```python
from build123d import *

# Parameters (mm, degrees)
SKETCH022_R             = 2.5
PAD022_DEPTH            = 10
SKETCH023_R             = 1.5
PAD023_DEPTH            = 10
SKETCH024_W             = 8
SKETCH024_H             = 14
PAD024_DEPTH            = 10
SKETCH025_W             = 5
SKETCH025_H             = 2
PAD025_DEPTH            = 10
BODY009_PLACEMENT_ANGLE = 90


with BuildPart() as part:
    # Sketch022 → Pad022 (new body)
    with BuildSketch(Plane.XZ):
        Circle(SKETCH022_R)
    extrude(amount=PAD022_DEPTH)

    # Sketch023 (on Face3 of Pad022) → Pad023 (join)
    with BuildSketch(Plane.XZ.offset(10)):
        Circle(SKETCH023_R)
    extrude(amount=PAD023_DEPTH)

    # Sketch024 (on Face2 of Pad023) → Pad024 (join)
    with BuildSketch(Plane(origin=(0, 0, 0), x_dir=(1, 0, 0), z_dir=(0, 1, 0))):
        Rectangle(SKETCH024_W, SKETCH024_H)
    extrude(amount=PAD024_DEPTH)

    # Sketch025 (on Face5 of Pad024) → Pad025 (join)
    with BuildSketch(Plane(origin=(0, 10, 0), x_dir=(1, 0, 0), z_dir=(0, 1, 0))):
        with Locations((0, 4.5)):
            Rectangle(SKETCH025_W, SKETCH025_H)
        Rectangle(SKETCH025_W, SKETCH025_H)
        with Locations((0, -4.5)):
            Rectangle(SKETCH025_W, SKETCH025_H)
    extrude(amount=PAD025_DEPTH)


with BuildPart() as part_1:
    # Body009 placement: moved
    add(part.part.moved(Location((-26, 13.5, 119))).rotate(Axis((-26, 13.5, 119), (-1, 0, 0)), BODY009_PLACEMENT_ANGLE))


solid = part_1.part
```
Verification items for the finished model (mm, model axes). A direction names the side the tool comes from. Coordinates: 2 decimals unless noted, no trailing zeros. Loops run counter-clockwise (first coordinate to the right, second up) from the corner with the lowest first, then second, coordinate; pieces in that order, holes last. Notation, with made-up numbers: (33.5, 44) -> (66.5, 44) arc R18 ccw to (66.5, 61) -> close; hole circle Ø5 at (51.25, 53). An arc over 180 degrees is marked (long way). Put each result on its own line as item: value.
1. Section check B-B, the plane y = 18. Record the boundary of the cut face in (x, z).
Result set:
outline: (-30, 109) -> (-28.5, 109) -> (-28.5, 99) -> (-23.5, 99) -> (-23.5, 109) -> (-22, 109) -> (-22, 119) -> (-30, 119) -> close
2. Section check A-A, the plane z = 103. Record the boundary of the cut face in (x, y), then the cut area to 3 significant figures.
Result set:
outline: (-28.5, 8) -> (-23.5, 8) -> (-23.5, 10) -> (-28.5, 10) -> close; (-28.5, 12.5) -> (-23.5, 12.5) -> (-23.5, 14.5) -> (-28.5, 14.5) -> close; (-28.5, 17) -> (-23.5, 17) -> (-23.5, 19) -> (-28.5, 19) -> close
area: 30.0 mm^2
3. Section check D-D, the plane z = 128. Record the boundary of the cut face in (x, y).
Result set:
outline: circle Ø5 at (-26, 13.5)
4. Thickness scan on line 1 (Y direction, x = -26, z = 107); line 2 (Z direction, x = -27.25, y = 15); line 3 (Z direction, x = -22.75, y = 18.75). Record the ranges inside material, lowest first.
Result set:
line 1: y = 8 to 10, 12.5 to 14.5, 17 to 19
line 2: z = 109 to 129
line 3: z = 109 to 119
5. Gauge pin test, flat ends, axial feed: P1, Ø1.5, axis at x = -26, z = 103, coming from the -Y side; P2, Ø0.6, axis at y = 14, z = 103.5, coming from the +X side; P3, Ø1.5, axis at x = -25, z = 104.5, coming from the +Y side. Record the tip position at first contact, or that the pin passes through.
Result set:
P1: stops at y = 8
P2: stops at x = -23.5
P3: stops at y = 19
6. Section check C-C, the plane x = -25.5. Record the boundary of the cut face in (y, z), then the cut area to 3 significant figures.
Result set:
outline: (6.5, 109) -> (8, 109) -> (8, 99) -> (10, 99) -> (10, 109) -> (12.5, 109) -> (12.5, 99) -> (14.5, 99) -> (14.5, 109) -> (17, 109) -> (17, 99) -> (19, 99) -> (19, 109) -> (20.5, 109) -> (20.5, 119) -> (15.95, 119) -> (15.95, 129) -> (14.91, 129) -> (14.91, 139) -> (12.09, 139) -> (12.09, 129) -> (11.05, 129) -> (11.05, 119) -> (6.5, 119) -> close
area: 277 mm^2
7. Mould release check, pull along Y, two halves, no side actions. Record for faces 6 (the face through (-26, 17, 104)), 7 (the face through (-26, 15, 109)), 8 (the face through (-27.5, 13.57, 133.93)), 9 (the face through (-25, 12, 129)): pulls with the +Y half, pulls with the -Y half, needs draft (parallel to the pull), parting line crosses it, or undercut.
Result set:
face 6: undercut
face 7: undercut
face 8: parting line crosses it
face 9: needs draft
8. Tool access check on faces 1 (the face through (-28.5, 9, 104)), 2 (the face through (-26, 8, 104)), 3 (the face through (-26, 14.5, 104)), 4 (the face through (-22, 14, 114)), 5 (the face through (-23.5, 18, 104)). Record the directions out of +Z, -Z, +X, -X, +Y, -Y that give a thin tool (end or side, any length) a straight path to the whole face; none if there is none.
Result set:
face 1: -Z, -X, +Y, -Y
face 2: -Z, +X, -X, -Y
face 3: -Z, +X, -X
face 4: +Z, -Z, +X, +Y, -Y
face 5: -Z, +X, +Y, -Y
